```python
from build123d import *

# Parameters (mm, degrees)
SKETCH1_W           = 76.2
SKETCH1_H           = 127
BOSS_EXTRUDE1_DEPTH = 6.35
CAVITY1_START       = -44.45
CAVITY1_OUTLINE_W   = 6.35
CAVITY1_OUTLINE_H   = 6.35
CAVITY1_DEPTH       = 12.7
CAVITY1_START_2     = -19.05
CAVITY1_2_OUTLINE_W = 6.35
CAVITY1_2_OUTLINE_H = 6.35
CAVITY1_2_DEPTH     = 12.7
CAVITY1_START_3     = 6.35
CAVITY1_3_OUTLINE_W = 6.35
CAVITY1_3_OUTLINE_H = 6.35
CAVITY1_3_DEPTH     = 12.7


# Read off the part's stored shape, not the designer's step: Cavity1
with BuildPart() as part:
    # Sketch1 → Boss-Extrude1 (new body)
    with BuildSketch(Plane.XY):
        with Locations((-6.35, -63.5)):
            Rectangle(SKETCH1_W, SKETCH1_H)
    extrude(amount=-BOSS_EXTRUDE1_DEPTH)

    # Cavity1 outline → Cavity1 (cut)
    with BuildSketch(Plane.YZ.offset(CAVITY1_START)):
        with Locations((-123.825, -3.175)):
            Rectangle(CAVITY1_OUTLINE_W, CAVITY1_OUTLINE_H)
        with Locations((-3.175, -3.175)):
            Rectangle(CAVITY1_OUTLINE_W, CAVITY1_OUTLINE_H)
    extrude(amount=CAVITY1_DEPTH, mode=Mode.SUBTRACT)

    # Cavity1 2 outline → Cavity1 2 (cut)
    with BuildSketch(Plane.YZ.offset(CAVITY1_START_2)):
        with Locations((-123.825, -3.175)):
            Rectangle(CAVITY1_2_OUTLINE_W, CAVITY1_2_OUTLINE_H)
        with Locations((-3.175, -3.175)):
            Rectangle(CAVITY1_2_OUTLINE_W, CAVITY1_2_OUTLINE_H)
    extrude(amount=CAVITY1_2_DEPTH, mode=Mode.SUBTRACT)

    # Cavity1 3 outline → Cavity1 3 (cut)
    with BuildSketch(Plane.YZ.offset(CAVITY1_START_3)):
        with Locations((-123.825, -3.175)):
            Rectangle(CAVITY1_3_OUTLINE_W, CAVITY1_3_OUTLINE_H)
        with Locations((-3.175, -3.175)):
            Rectangle(CAVITY1_3_OUTLINE_W, CAVITY1_3_OUTLINE_H)
    extrude(amount=CAVITY1_3_DEPTH, mode=Mode.SUBTRACT)


solid = part.part
```
The listing builds one solid part. Answer for the finished solid, in the listing's coordinates (mm). A direction names the side the tool comes from. Coordinates: 2 decimals unless noted, no trailing zeros. Loops run counter-clockwise (first coordinate to the right, second up) from the corner with the lowest first, then second, coordinate; pieces in that order, holes last. Notation, with made-up numbers: (30, 61.25) - (62, 61.25) arc R24 cw to (62, 71.25) - close; hole circle Ø3 at (-25, 82.25). An arc over 180 degrees is marked (long way). Use a Markdown table: item, result. Add a question column.
1) Given pin 1 (12 mm diameter, centred on x = -22.5, y = -92, fed in from +Z); pin 2 (1.9 mm diameter, centred on x = 15.5, z = -3.5, fed in from +Y); pin 3 (1.9 mm diameter, centred on x = -11.5, z = -2.5, fed in from -Y); pin 4 (3 mm diameter, centred on y = -122.5, z = -2, fed in from -X), each flat-ended and moving along its own axis, determine where each tip first touches the part or whether it passes through.
2) The part is cut by section B-B, the plane x = 17. Give the vertices of the cut face in (y, z), and give its area (3 significant figures).
3) Find the intervals of material crossed by line 1 (Y direction, x = -7, z = -1.75), in increasing order.
4) The part is cut by section A-A, the plane z = -4.25. Give the vertices of the cut face in (x, y), and give its area (3 significant figures).
5) The mould has two halves that part along X. Classify faces 1 (the flat face through (13, -6.35, -3)), 2 (the flat face through (0, 0, -3)), 3 (the flat face through (31.75, -64, -3)), 4 (the flat face through (19.05, -124, -3)): released by +X, released by -X, zero draft, split by the parting line, or undercut.
6) For faces 5 (the flat face through (6.35, -3, -3)), 6 (the flat face through (-38, -6.35, -3)), 7 (the flat face through (13, -120.65, -3)), determine the directions among +Z, -Z, +X, -X, +Y, -Y from which every point of the face is accessible in a straight line to the end or side of a thin tool.
Here are the results:
| question | item | result |
|---|---|---|
| 1 | pin 1 | stops at z = 0 |
| 1 | pin 2 | stops at y = -6.35 |
| 1 | pin 3 | stops at y = -120.65 |
| 1 | pin 4 | stops at x = -31.75 |
| 2 | outline | (-120.65, -6.35) - (-6.35, -6.35) - (-6.35, 0) - (-120.65, 0) - close |
| 2 | area | 726 mm^2 |
| 3 | line 1 | y = -120.65 to -6.35 |
| 4 | outline | (-44.45, -120.65) - (-31.75, -120.65) - (-31.75, -127) - (-19.05, -127) - (-19.05, -120.65) - (-6.35, -120.65) - (-6.35, -127) - (6.35, -127) - (6.35, -120.65) - (19.05, -120.65) - (19.05, -127) - (31.75, -127) - (31.75, 0) - (19.05, 0) - (19.05, -6.35) - (6.35, -6.35) - (6.35, 0) - (-6.35, 0) - (-6.35, -6.35) - (-19.05, -6.35) - (-19.05, 0) - (-31.75, 0) - (-31.75, -6.35) - (-44.45, -6.35) - close |
| 4 | area | 9,190 mm^2 |
| 5 | face 1 | undercut |
| 5 | face 2 | zero draft |
| 5 | face 3 | released by +X |
| 5 | face 4 | undercut |
| 6 | face 5 | +Z, -Z, +Y |
| 6 | face 6 | +Z, -Z, -X, +Y |
| 6 | face 7 | +Z, -Z, -Y |
